Read the model definition and answer for the solid it produces. Units are mm, in the model's axes. Round coordinates to 2 decimals unless told otherwise and drop trailing zeros. Order: outer loops, then holes, each group sorted by start corner. A loop starts at its lowest first (then second) coordinate and runs counter-clockwise, first axis right, second up. Notation, with made-up numbers: (50.25, 21.25) -> (77.25, 21.25) arc R17 cw to (77.25, 52.25) -> close; hole circle Ø3 at (58.25, 42). An arc over 180 degrees is marked (long way). Use a Markdown table: item, result. Add a question column.
1. Section A-A, the plane z = 19.5 is taken. Give the vertices of the cut face in (x, y), then the cut area to 3 significant figures.
2. Consider L1, parallel to X at y = 0, z = 19.25; L2, parallel to X at y = -5, z = 13.75; L3, parallel to Y at x = 242, z = 16.25. Determine where each line is inside the solid, lowest interval first. Write a range as [from, to].
3. Section B-B, the plane x = 242 is taken. Give the vertices of the cut face in (y, z), then the cut area to 3 significant figures.
4. The mould has two halves that part along X. Classify faces 1 (the face through (-247.952, -4.564, 18.662)), 2 (the face through (262, 0, 19)), 3 (the face through (-258.58, 8.89, 18.66)): +X half, -X half, draft (parallel to the pull), parting line (faces both ways), or undercut.
5. Given pin 1 (5 mm diameter, centred on y = 5, z = 18, fed in from -X); pin 2 (5 mm diameter, centred on y = -6, z = 16, fed in from -X), each flat-ended and moving along its own axis, determine where each tip first touches the part or whether it passes through.
```python
from build123d import *

# Parameters (mm, degrees)
SKETCH1_R               = 7.5
BOSS_EXTRUDE2_DEPTH     = 25
CUT_EXTRUDE1_DEPTH      = 525.744938041
CUT_EXTRUDE1_DEPTH_BACK = 525.744938041
SKETCH2_W               = 12.5
SKETCH2_H               = 25


with BuildPart() as part:
    # Sketch1 → Boss-Extrude2 (new body)
    with BuildSketch(Plane.XY):
        with BuildLine():
            Line((-250, 12.5), (262, 12.5))
            Line((262, 12.5), (262, -12.5))
            Line((262, -12.5), (-250, -12.5))
            ThreePointArc((-250, -12.5), (-258.485281374, -8.985281374), (-262, -0.5))
            Line((-262, -0.5), (-262, 0.5))
            ThreePointArc((-262, 0.5), (-258.485281374, 8.985281374), (-250, 12.5))
        make_face()
        with Locations((-242, 0)):
            Circle(SKETCH1_R, mode=Mode.SUBTRACT)
        with Locations((242, 0)):
            Circle(SKETCH1_R, mode=Mode.SUBTRACT)
    extrude(amount=BOSS_EXTRUDE2_DEPTH)

    # Sketch2 → Cut-Extrude1 (cut, two sides: drawn at the far end of the back side and taken through both)
    with BuildSketch(Plane(origin=(262, 0, 0), x_dir=(0, 0, -1), z_dir=(1, 0, 0)).offset(-CUT_EXTRUDE1_DEPTH_BACK)):
        with Locations((-6.25, 0)):
            Rectangle(SKETCH2_W, SKETCH2_H)
    extrude(amount=CUT_EXTRUDE1_DEPTH + CUT_EXTRUDE1_DEPTH_BACK, mode=Mode.SUBTRACT)


solid = part.part
```
Verdict:
| question | item | result |
|---|---|---|
| 1 | outline | (-262, -0.5) arc R12 ccw to (-250, -12.5) -> (262, -12.5) -> (262, 12.5) -> (-250, 12.5) arc R12 ccw to (-262, 0.5) -> close; hole circle Ø15 at (-242, 0); hole circle Ø15 at (242, 0) |
| 1 | area | 12,700 mm2 |
| 2 | L1 | x = [-262, -249.5], [-234.5, 234.5], [249.5, 262] |
| 2 | L2 | x = [-261.12, -247.59], [-236.41, 236.41], [247.59, 262] |
| 2 | L3 | y = [-12.5, -7.5], [7.5, 12.5] |
| 3 | outline | (-12.5, 12.5) -> (-7.5, 12.5) -> (-7.5, 25) -> (-12.5, 25) -> close; (7.5, 12.5) -> (12.5, 12.5) -> (12.5, 25) -> (7.5, 25) -> close |
| 3 | area | 125 mm2 |
| 4 | face 1 | undercut |
| 4 | face 2 | +X half |
| 4 | face 3 | -X half |
| 5 | pin 1 | stops at x = -261.83 |
| 5 | pin 2 | stops at x = -261.62 |
